```python
from build123d import *

# Parameters (mm, degrees)
BOSS_EXTRUDE1_DEPTH = 30
SKETCH2_R           = 25
SKETCH2_R_2         = 30
CUT_EXTRUDE1_DEPTH  = 527.798524366
SKETCH4_R           = 40
SKETCH4_R_2         = 30
BOSS_EXTRUDE3_DEPTH = 10
SCALE1_SCALE        = 0.1


with BuildPart() as part:
    # Sketch1 → Boss-Extrude1 (new body)
    with BuildSketch(Plane.XY):
        with BuildLine():
            ThreePointArc((-267.733324074, 386.480114093), (-317.733324074, 336.480114093), (-267.733324074, 286.480114093))
            add(Edge.make_bspline(
                [(-267.733324074, 286.480114093), (-61.536299878, 365.758634067), (152.142574227, 266.270803333)],
                knots=[0, 0, 0, 1, 1, 1], degree=2))
            ThreePointArc((152.142574227, 266.270803333), (212.142574227, 326.270803333), (152.142574227, 386.270803333))
            add(Edge.make_bspline(
                [(-267.733324074, 386.480114093), (-58.376892778, 451.86591416), (152.142574227, 386.270803333)],
                knots=[0, 0, 0, 1, 1, 1], degree=2))
        make_face()
    extrude(amount=BOSS_EXTRUDE1_DEPTH)

    # Sketch2 → Cut-Extrude1 (cut, through all)
    with BuildSketch(Plane.XY):
        with Locations((-267.733324074, 336.480114093)):
            Circle(SKETCH2_R)
        with Locations((152.142574227, 326.270803333)):
            Circle(SKETCH2_R_2)
    extrude(amount=CUT_EXTRUDE1_DEPTH, mode=Mode.SUBTRACT)

    # Sketch4 → Boss-Extrude3 (add)
    with BuildSketch(Plane.XY.offset(30)):
        with Locations((152.142574227, 326.270803333)):
            Circle(SKETCH4_R)
        with Locations((152.142574227, 326.270803333)):
            Circle(SKETCH4_R_2, mode=Mode.SUBTRACT)
    extrude(amount=BOSS_EXTRUDE3_DEPTH)


with BuildPart() as part_1:
    # Scale1: scaled about (-43.370651933, 353.535569424, 15.302961692)
    add(part.part.scale(SCALE1_SCALE).moved(Location((-39.03358674, 318.182012482, 13.772665523))))


solid = part_1.part
```
The model under review builds one solid part; all positions refer to its coordinate system, in mm. A direction names the side the tool comes from. Round coordinates to 2 decimals unless told otherwise and drop trailing zeros. Loops run counter-clockwise (first coordinate to the right, second up) from the corner with the lowest first, then second, coordinate; pieces in that order, holes last.
Item 1: Mouldability with a two-part tool opening along Y and no side actions: class faces 1 (the face through (-17.82, 350.68, 15.25)), 2 (the face through (-64.653, 349.612, 15.252)), 3 (the face through (-45, 354, 16.773)), 4 (the face through (-22.435, 348.148, 15.745)) as released by +Y, released by -Y, zero draft, split by the parting line, or undercut.
Determined:
face 1: split by the parting line
face 2: undercut
face 3: zero draft
face 4: undercut
Item 2: For line 1 (X direction, y = 352.75, z = 16.45); line 2 (Z direction, x = -50, y = 355.5); line 3 (Y direction, x = -67.5, z = 15.9), list the stretches that pass through material, from the lowest coordinate up.
Determined:
line 1: x = -70.72 to -68.13, -63.48 to -26.11, -21.53 to -18.14
line 2: z = 13.77 to 16.77
line 3: y = 347.13 to 349.99, 353.67 to 356.53
Item 3: Take a section at A-A (y = 348.5). Give the number of separate pieces and of enclosed holes in the cut face, then the cut area to 3 significant figures.
Determined:
separate pieces: 3
enclosed holes: 0
area: 64.2 mm2
Item 4: For faces 5 (the face through (-45, 354, 13.773)), 6 (the face through (-21.974, 347.26, 17.266)), list the 3-axis set-ups (+Z, -Z, +X, -X, +Y, -Y) from which the entire face can be reached by the end or side of a thin tool; tool diameter is ignored.
Determined:
face 5: -Z, +X, -X, +Y, -Y
face 6: +Z
Item 5: Clearance check with flat-ended pins moving along their axes: pin 1 Ø2 at (y, z) = (350.5, 16) entering from -X; pin 2 Ø1.5 at (x, z) = (-38.5, 17) entering from -Y; pin 3 Ø1.5 at (x, y) = (-45.5, 358) entering from +Z. State where each tip first meets the part, or that it passes through.
Determined:
pin 1: stops at x = -70.8
pin 2: stops at y = 349.42
pin 3: stops at z = 16.77
Item 6: Take a section at C-C (y = 356). Write out the cut boundary in (x, z).
Determined:
outline: (-68.57, 13.77) - (-20.81, 13.77) - (-20.81, 16.77) - (-68.57, 16.77) - close
